from build123d import *

# Parameters (mm, degrees)
F3_DEPTH     = 7.62
F4_DEPTH     = 4.318
F1_W         = 86.36
F1_H         = 55.88
F5_DEPTH     = 3.81
F6_W         = 6.2699629925
F6_H         = 43.1555788964
F7_DEPTH     = 4.572
F8_R         = 5.08
F9_T1_DEPTH  = 135.8469622158
F10_R        = 5.08
F11_T1_DEPTH = 135.8469622158


# Not quite as in the source:
# - a fillet or chamfer that OpenCascade refuses, or shapes differently, is made with other operations: its cross-section is extruded or revolved along the edge and cut away or added


with BuildPart() as f3:
    # F2 (on Front) → F3 (new body)
    with BuildSketch(Plane.XZ):
        Polygon((-6.2699629925, 72.1773862183), (-6.2699629925, 59.4773862183), (-6.2699629925, -68.8154984593), (-6.2699629925, -81.5154984593), (91.4769992232, -81.5154984593), (91.4769992232, -68.8154984593), (91.4769992232, 59.4773862183), (91.4769992232, 72.1773862183), align=None)
    extrude(amount=F3_DEPTH)

    # F0 (on Front) → F4 (cut)
    with BuildSketch(Plane.XZ):
        Polygon((0, 53.34), (0, 0), (66.5871798992, 0), (70.5303996801, 0), (78.1503996801, 0), (78.1503996801, 53.34), (70.5303996801, 53.34), (64.516, 53.34), align=None)
    extrude(amount=F4_DEPTH, mode=Mode.SUBTRACT)

    # F1 (on Front) → F5 (cut)
    with BuildSketch(Plane.XZ):
        with Locations((43.18, -36.3771444535)):
            Rectangle(F1_W, F1_H)
    extrude(amount=F5_DEPTH, mode=Mode.SUBTRACT)

    # F6 (on face) → F7 (cut)
    with BuildSketch(Plane(origin=(0, 0, 0), x_dir=(-1, 0, 0), z_dir=(0, 1, 0))):
        with Locations((3.1349814963, 28.3439913765)):
            Rectangle(F6_W, F6_H)
    extrude(amount=-F7_DEPTH, mode=Mode.SUBTRACT)

    # F8
    f8_edges = [f3.edges().sort_by_distance(p)[0] for p in [
        (42.603518, -7.62, -81.515498),
    ]]
    fillet(f8_edges, radius=F8_R)

    # F9: fillet of radius 12.7 on 1 edges, made by hand

    # F9_s2 → F9_t1 (cut)
    with BuildSketch(Plane.YZ.offset(-25.3199629925)):
        with BuildLine():
            ThreePointArc((-2.54, -81.5154984593), (-0.6517221148, -77.9115910878), (0, -73.8954984593))
            Line((0, -73.8954984593), (0, -81.5154984593))
            Line((0, -81.5154984593), (-2.54, -81.5154984593))
        make_face()
    extrude(amount=F9_T1_DEPTH, mode=Mode.SUBTRACT)

    # F10
    f10_edges = [f3.edges().sort_by_distance(p)[0] for p in [
        (42.603518, -7.62, 72.177386),
    ]]
    fillet(f10_edges, radius=F10_R)

    # F11: fillet of radius 12.7 on 1 edges, made by hand

    # F11_s2 → F11_t1 (cut)
    with BuildSketch(Plane.YZ.offset(-25.3199629925)):
        with BuildLine():
            ThreePointArc((-2.54, 72.1773862183), (-0.6517221148, 68.5734788467), (0, 64.5573862183))
            Line((0, 64.5573862183), (0, 72.1773862183))
            Line((0, 72.1773862183), (-2.54, 72.1773862183))
        make_face()
    extrude(amount=F11_T1_DEPTH, mode=Mode.SUBTRACT)


solid = f3.part
CAD build for the part. Positions are in the model's coordinates, mm. A direction names the side the tool comes from. Coordinates: 2 decimals unless noted, no trailing zeros. Loops run counter-clockwise (first coordinate to the right, second up) from the corner with the lowest first, then second, coordinate; pieces in that order, holes last. Notation, with made-up numbers: (29.25, 4.25) - (69.25, 4.25) arc R9 cw to (69.25, 17.25) - close; hole circle Ø8 at (44.5, 42). An arc over 180 degrees is marked (long way). Write item = value, one per line. Start each with the question number.
Q1. Flat gauge pins, fed straight in: pin 1 Ø1.4 at (x, y) = (-1.5, -1) entering from -Z; pin 2 Ø4 at (x, y) = (73, -6.5) entering from +Z; pin 3 Ø4.5 at (x, y) = (22, -2) entering from -Z; pin 4 Ø3 at (x, z) = (71, -29) entering from +Y. Where does each tip first touch, or does it go through?
Q2. Cut at C-C, the plane y = -1.25. List the corners of the cut face in (x, z), then the cut area to 3 significant figures.
Q3. Drill centre lines: L1, parallel to Z at x = 53.5, y = -3.5; L2, parallel to Z at x = 78, y = -3.75; L3, parallel to X at y = -1.25, z = -43.5. Where is each one in solid material? Low to high.
Q4. Cut at A-A, the plane x = 83. List the corners of the cut face in (y, z), then the cut area to 3 significant figures.
Q5. Cut at D-D, the plane x = 18. List the corners of the cut face in (y, z).
Q6. Pull direction X, two halves, no side cores. Call faces 1 (the flat face through (-6.27, -4, -4)), 2 (the flat face through (43, -2, -64.317)), 3 (the flat face through (42, -7.62, -4)), 4 (the flat face through (40, -2, 53.34)): pulls with the +X half, pulls with the -X half, needs draft (parallel to the pull), parting line crosses it, or undercut.
Q7. Cut at B-B, the plane z = -50.5. List the corners of the cut face in (x, y).
Q8. Which spindle directions (+Z, -Z, +X, -X, +Y, -Y) get a long thin tool onto all of the face, cutting with end or side? Do faces 5 (the flat face through (78.15, -2, 26)), 6 (the flat face through (-3, -2, 6.766)), 7 (the cylindrical face through (43.29, -6.09, -80.07)). Say none if no direction does.
Computed:
q1.pin_1 = -80.24
q1.pin_2 = 71.78
q1.pin_3 = -81.52
q1.pin_4 = -3.81
q2.outline = (-6.27, -79.39) - (91.48, -79.39) - (91.48, 70.05) - (-6.27, 70.05) - (-6.27, 49.92) - (0, 49.92) - (0, 53.34) - (78.15, 53.34) - (78.15, 0) - (0, 0) - (0, 6.77) - (-6.27, 6.77) - close; hole (0, -64.32) - (86.36, -64.32) - (86.36, -8.44) - (0, -8.44) - close
q2.area = 5,340 mm²
q3.L1 = -81.42 to -64.32, -8.44 to 0, 53.34 to 72.09
q3.L2 = -81.37 to -64.32, -8.44 to 0, 53.34 to 72.03
q3.L3 = -6.27 to 0, 86.36 to 91.48
q4.outline = (-7.62, -76.44) arc R5.08 ccw to (-2.54, -81.52) arc R12.7 ccw to (0, -73.9) - (0, -64.32) - (-3.81, -64.32) - (-3.81, -8.44) - (0, -8.44) - (0, 64.56) arc R12.7 ccw to (-2.54, 72.18) arc R5.08 ccw to (-7.62, 67.1) - close
q4.area = 935 mm²
q5.outline = (-7.62, -76.44) arc R5.08 ccw to (-2.54, -81.52) arc R12.7 ccw to (0, -73.9) - (0, -64.32) - (-3.81, -64.32) - (-3.81, -8.44) - (0, -8.44) - (0, 0) - (-4.32, 0) - (-4.32, 53.34) - (0, 53.34) - (0, 64.56) arc R12.7 ccw to (-2.54, 72.18) arc R5.08 ccw to (-7.62, 67.1) - close
q6.face_1 = pulls with the -X half
q6.face_2 = undercut
q6.face_3 = needs draft
q6.face_4 = undercut
q7.outline = (-6.27, -7.62) - (91.48, -7.62) - (91.48, 0) - (86.36, 0) - (86.36, -3.81) - (0, -3.81) - (0, 0) - (-6.27, 0) - close
q8.face_5 = +Y
q8.face_6 = -X, +Y
q8.face_7 = -Z, +X, -X, -Y
